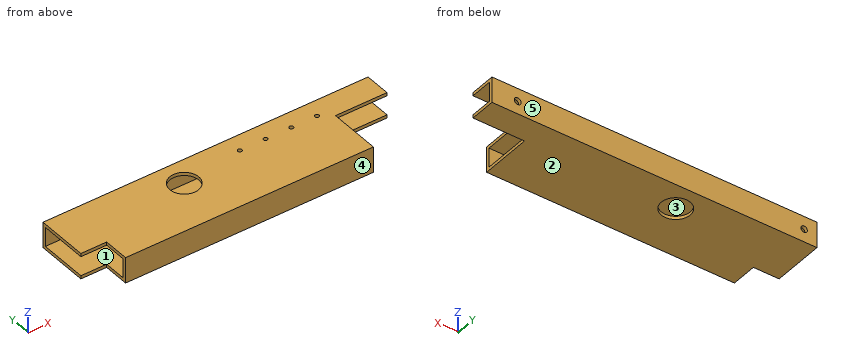
from build123d import *

# Parameters (mm, degrees)
BOSS_EXTRUDE1_DEPTH         = 12.7
F_1_4_0_25_DIAMETER_HOLE1_D = 6.35
CUT_EXTRUDE1_DEPTH          = 580.243923145
SKETCH8_R                   = 14.2875
CUT_EXTRUDE2_DEPTH          = 293.531067795
F_10_32_TAPPED_HOLE1_D      = 4.0386
F_10_32_TAPPED_HOLE1_DEPTH  = 13.716
F_10_32_TAPPED_HOLE1_TIP    = 1.213317848
SKETCH11_W                  = 257.175
SKETCH11_H                  = 76.2
CUT_EXTRUDE3_DEPTH          = 293.531067795
SKETCH13_W                  = 50.8
SKETCH13_H                  = 50.8
CUT_EXTRUDE5_DEPTH          = 293.531067795
F_1_4_CLEARANCE_HOLE1_D     = 6.7564


with BuildPart() as part:
    # Sketch1 → Boss-Extrude1 (new, symmetric)
    with BuildSketch(Plane.XY):
        Polygon((-288.925, 38.1), (-288.925, -12.7), (-263.525, -12.7), (-263.525, -38.1), (263.525, -38.1), (263.525, -12.7), (288.925, -12.7), (288.925, 38.1), align=None)
    extrude(amount=BOSS_EXTRUDE1_DEPTH, both=True)

    # 1/4 (0.25) Diameter Hole1 (through all)
    with Locations(Plane(origin=(0, 38.1, 0), x_dir=(1, 0, 0), z_dir=(0, 1, 0))):
        with Locations((-276.225, 0), (276.225, 0)):
            Hole(F_1_4_0_25_DIAMETER_HOLE1_D / 2)

    # Sketch5 → Cut-Extrude1 (cut, through all)
    with BuildSketch(Plane(origin=(288.925, 0, 0), x_dir=(0, 0, -1), z_dir=(1, 0, 0))):
        Polygon((9.525, -12.7), (9.525, 34.925), (-9.525, 34.925), (-9.525, -12.7), (-9.525, -34.925), (9.525, -34.925), align=None)
    extrude(amount=-CUT_EXTRUDE1_DEPTH, mode=Mode.SUBTRACT)

    # Sketch8 → Cut-Extrude2 (cut, through all)
    with BuildSketch(Plane.XY.offset(12.7)):
        with Locations((-168.275, 12.7)):
            Circle(SKETCH8_R)
        with Locations((168.275, 12.7)):
            Circle(SKETCH8_R)
    extrude(amount=-CUT_EXTRUDE2_DEPTH, mode=Mode.SUBTRACT)

    # #10-32 Tapped Hole1
    with Locations(Plane.XY.offset(12.7)):
        with Locations((-107.315, 21.082), (-81.915, 21.082), (-56.515, 21.082), (-31.115, 21.082)):
            Hole(F_10_32_TAPPED_HOLE1_D / 2, depth=F_10_32_TAPPED_HOLE1_DEPTH)
            with Locations((0, 0, -(F_10_32_TAPPED_HOLE1_DEPTH + F_10_32_TAPPED_HOLE1_TIP / 2))):  # 118° drill point
                Cone(0, F_10_32_TAPPED_HOLE1_D / 2, F_10_32_TAPPED_HOLE1_TIP, mode=Mode.SUBTRACT)

    # Sketch11 → Cut-Extrude3 (cut, through all)
    with BuildSketch(Plane.XY.offset(12.7)):
        with Locations((160.3375, 0)):
            Rectangle(SKETCH11_W, SKETCH11_H)
    extrude(amount=-CUT_EXTRUDE3_DEPTH, mode=Mode.SUBTRACT)

    # Sketch13 → Cut-Extrude5 (cut, through all)
    with BuildSketch(Plane.XY.offset(12.7)):
        with Locations((6.35, -12.7)):
            Rectangle(SKETCH13_W, SKETCH13_H)
    extrude(amount=-CUT_EXTRUDE5_DEPTH, mode=Mode.SUBTRACT)

    # 1/4 Clearance Hole1 (through all)
    with Locations(Plane(origin=(0, 38.1, 0), x_dir=(1, 0, 0), z_dir=(0, 1, 0))):
        with Locations((6.35, 0)):
            Hole(F_1_4_CLEARANCE_HOLE1_D / 2)


solid = part.part
Part model, mm, in its own coordinate system. Face numbers are marked on the shaded views. A direction names the side the tool comes from. Give positions to 0.01 mm unless a question says otherwise; leave off trailing zeros. Loops run counter-clockwise (first coordinate to the right, second up) from the corner with the lowest first, then second, coordinate; pieces in that order, holes last. Notation, with made-up numbers: (-14.75, 21) -> (32.25, 21) arc R19 cw to (32.25, 40) -> close; hole circle Ø11 at (-25, 85.25). An arc over 180 degrees is marked (long way). Write each question's results on one line, items separated by ' | '. Start each with the question number.
Q1. Band-saw the part on B-B on y = -9. List the corners of the cut face in (x, z) (3 decimals), plus the area to 3 significant figures.
Q2. Band-saw the part on C-C on z = 0. List the corners of the cut face in (x, y) (3 decimals), plus the area to 3 significant figures.
Q3. Which spindle directions (+Z, -Z, +X, -X, +Y, -Y) get a long thin tool onto all of the face, cutting with end or side? Do the marked faces 1 and 2. Say none if no direction does.
Q4. Wall check: L1, parallel to Y at x = -72.5, z = -5.75 (3 decimals); L2, parallel to Z at x = -154, y = 20 (3 decimals); L3, parallel to X at y = -30, z = -10.5 (3 decimals). Give the ranges that are in metal, low to high.
Q5. Pull direction Y, two halves, no side cores. Call the marked faces 3, 4 and 5: +Y half, -Y half, draft (parallel to the pull), parting line (faces both ways), or undercut.
Q6. Pin check, flat tips, straight feed: P1, Ø2, axis at y = -21, z = 10, coming from the +X side; P2, Ø6.5, axis at x = -31.115, y = 21.082, coming from the +Z side; P3, Ø2.5, axis at x = -273, z = 10.5, coming from the -Y side; P4, Ø9, axis at x = 6.35, z = 0, coming from the -Y side (3 decimals). Stop position of each tip, or through.
Q7. Band-saw the part on D-D on x = -36.5. List the corners of the cut face in (y, z) (3 decimals).
Q8. Band-saw the part on A-A on x = 6.35. List the corners of the cut face in (y, z) (3 decimals), plus the area to 3 significant figures.
Results are:
1) outline: (-288.925, -12.7) -> (-19.05, -12.7) -> (-19.05, -9.525) -> (-288.925, -9.525) -> close; (-288.925, 9.525) -> (-19.05, 9.525) -> (-19.05, 12.7) -> (-288.925, 12.7) -> close | area: 1,710 mm²
2) outline: (-288.925, 34.925) -> (-279.4, 34.925) -> (-279.4, 38.1) -> (-288.925, 38.1) -> close; (-273.05, 34.925) -> (2.972, 34.925) -> (2.972, 38.1) -> (-273.05, 38.1) -> close; (-263.525, -38.1) -> (-19.05, -38.1) -> (-19.05, -34.925) -> (-263.525, -34.925) -> close; (9.728, 34.925) -> (31.75, 34.925) -> (31.75, 38.1) -> (9.728, 38.1) -> close | area: 1,750 mm²
3) face 1: +X, -X | face 2: -Z, +X, -X, +Y, -Y
4) L1: y = -38.1 to -34.925, 34.925 to 38.1 | L2: z = -12.7 to -9.525, 9.525 to 12.7 | L3: x = -263.525 to -19.05
5) face 3: undercut | face 4: -Y half | face 5: +Y half
6) P1: stops at x = -19.05 | P2: stops at z = 12.7 | P3: stops at y = -12.7 | P4: stops at y = 34.925
7) outline: (-38.1, -12.7) -> (38.1, -12.7) -> (38.1, 12.7) -> (-38.1, 12.7) -> close; hole (-34.925, -9.525) -> (34.925, -9.525) -> (34.925, 9.525) -> (-34.925, 9.525) -> close
8) outline: (12.7, -12.7) -> (38.1, -12.7) -> (38.1, -3.378) -> (34.925, -3.378) -> (34.925, -9.525) -> (12.7, -9.525) -> close; (12.7, 9.525) -> (34.925, 9.525) -> (34.925, 3.378) -> (38.1, 3.378) -> (38.1, 12.7) -> (12.7, 12.7) -> close | area: 200 mm²
